The model under review builds one solid part; all positions refer to its coordinate system, in mm. A direction names the side the tool comes from. Coordinates: 2 decimals unless noted, no trailing zeros. Write each loop counter-clockwise with the first axis right and the second up, starting at its lowest first coordinate (ties: lowest second). Pieces come first, ordered by that corner, then holes. Notation, with made-up numbers: (-23.5, 80) - (19.5, 80) arc R25 ccw to (19.5, 115) - close; hole circle Ø11 at (75, 80). An arc over 180 degrees is marked (long way). Use one line per item in the form item = value. Start each with the question number.
```python
from build123d import *

# Parameters (mm, degrees)
SKETCH1_W               = 58
SKETCH1_H               = 58
BOSS_EXTRUDE1_DEPTH     = 10
BOSS_EXTRUDE3_DEPTH     = 30.005
CIRPATTERN7_COUNT       = 4
CUT_EXTRUDE1_DEPTH      = 13
CUT_EXTRUDE1_DEPTH_BACK = 11
SKETCH8_R               = 1.75
CUT_EXTRUDE2_DEPTH      = 20
SKETCH9_R               = 3.665
CUT_EXTRUDE3_DEPTH      = 2.1


with BuildPart() as part:
    # Sketch1 → Boss-Extrude1 (new body)
    with BuildSketch(Plane(origin=(0, 0, 0), x_dir=(1, 0, 0), z_dir=(0, 1, 0))):
        Rectangle(SKETCH1_W, SKETCH1_H)
    extrude(amount=BOSS_EXTRUDE1_DEPTH)

    # Sketch2 → Boss-Extrude3 (add, symmetric)
    with BuildSketch(Plane.XY):
        with BuildLine():
            Line((29, 0), (29, 14))
            Line((29, 14), (40.244226325, 21.496150883))
            ThreePointArc((40.244226325, 21.496150883), (41.038974467, 21.871276079), (41.908326913, 22))
            Line((41.908326913, 22), (44, 22))
            Line((44, 22), (31, 0))
            Line((31, 0), (29, 0))
        make_face()
    boss_extrude3 = extrude(amount=BOSS_EXTRUDE3_DEPTH, both=True)

    # CirPattern7: Boss-Extrude3 ×4 about axis
    cirpattern7_axis = Axis((0, 0, 0), (0, 1, 0))
    for i in range(1, CIRPATTERN7_COUNT):
        add(boss_extrude3.rotate(cirpattern7_axis, i * 360 / CIRPATTERN7_COUNT))

    # Sketch7 → Cut-Extrude1 (cut, two sides)
    with BuildSketch(Plane(origin=(0, 10, 0), x_dir=(1, 0, 0), z_dir=(0, 1, 0))) as cut_extrude1_sk:
        with BuildLine():
            Line((21.84, 7), (54.527297937, 7))
            Line((54.527297937, 7), (54.527297937, -7))
            Line((54.527297937, -7), (21.84, -7))
            ThreePointArc((21.84, -7), (14.84, 0), (21.84, 7))
        make_face()
        with BuildLine():
            Line((7, -21.84), (7, -54.527297937))
            Line((7, -54.527297937), (-7, -54.527297937))
            Line((-7, -54.527297937), (-7, -21.84))
            ThreePointArc((-7, -21.84), (0, -14.84), (7, -21.84))
        make_face()
        with BuildLine():
            Line((-21.84, -7), (-54.527297937, -7))
            Line((-54.527297937, -7), (-54.527297937, 7))
            Line((-54.527297937, 7), (-21.84, 7))
            ThreePointArc((-21.84, 7), (-14.84, 0), (-21.84, -7))
        make_face()
        with BuildLine():
            Line((-7, 21.84), (-7, 54.527297937))
            Line((-7, 54.527297937), (7, 54.527297937))
            Line((7, 54.527297937), (7, 21.84))
            ThreePointArc((7, 21.84), (0, 14.84), (-7, 21.84))
        make_face()
    extrude(amount=CUT_EXTRUDE1_DEPTH, mode=Mode.SUBTRACT)
    extrude(cut_extrude1_sk.sketch, amount=-CUT_EXTRUDE1_DEPTH_BACK, mode=Mode.SUBTRACT)

    # Sketch8 → Cut-Extrude2 (cut)
    with BuildSketch(Plane(origin=(-225.294025085, 10, 60.777514946), x_dir=(0, 0, -1), z_dir=(0, 1, 0))):
        with Locations((74.91965057, -211.151889461)):
            Circle(SKETCH8_R)
        with Locations((74.91965057, -239.436160708)):
            Circle(SKETCH8_R)
        with Locations((46.635379323, -239.436160708)):
            Circle(SKETCH8_R)
    extrude(amount=-CUT_EXTRUDE2_DEPTH, mode=Mode.SUBTRACT)

    # Sketch9 → Cut-Extrude3 (cut)
    with BuildSketch(Plane(origin=(0, 10, 0), x_dir=(1, 0, 0), z_dir=(0, 1, 0))):
        with Locations((-14.142135624, 14.142135624)):
            Circle(SKETCH9_R)
        with Locations((14.142135624, -14.142135624)):
            Circle(SKETCH9_R)
        with Locations((14.142135624, 14.142135624)):
            Circle(SKETCH9_R)
    extrude(amount=-CUT_EXTRUDE3_DEPTH, mode=Mode.SUBTRACT)


solid = part.part
```
1. Take a section at A-A (z = 34.5). State the section outline as (x, y) points (3 decimals).
2. Take a section at B-B (x = 38.5). State the section outline as (y, z) points (3 decimals), plus the area to 3 significant figures.
3. For P1, Ø11, axis at x = -32.5, y = 16, coming from the -Z side; P2, Ø3, axis at x = -14.14, z = -14.14, coming from the -Y side; P3, Ø3, axis at x = -1, y = 3.5, coming from the +Z side; P4, Ø10, axis at x = 10, y = 6, coming from the -Z side, all flat-tipped, find the tip position at first contact; note any pin that passes through.
4. For faces 4 (the flat face through (30, 9, -7)), 5 (the cylindrical face through (16.112, 8.965, -17.232)), 6 (the flat face through (-37.59, 11.15, 18.34)), 7 (the flat face through (-7, 9, 31)), list the 3-axis set-ups (+Z, -Z, +X, -X, +Y, -Y) from which the entire face can be reached by the end or side of a thin tool; tool diameter is ignored.
5. For L1, parallel to X at y = 16.5, z = 38 (3 decimals); L2, parallel to X at y = 9.75, z = -14.5, list the stretches that pass through material, from the lowest coordinate up.
6. Take a section at C-C (y = 12.75). Count the separate pieces of the cut face and the enclosed holes in it, plus the area to 3 significant figures.
7. The part is to be moulded in two halves that separate along Z. For faces 1 (the flat face through (-36, 14, -30.005)), 2 (the cylindrical face through (-12.17, 8.96, -17.23)), 3 (the flat face through (7, 9, -31)), say which applies: released by +Z, released by -Z, zero draft, split by the parting line, or undercut.
Returned:
q1.outline = (-30.005, 5.923) - (-7, 5.923) - (-7, 17.667) - (-30.005, 17.667) - close; (7, 5.923) - (30.005, 5.923) - (30.005, 17.667) - (7, 17.667) - close
q2.outline = (12.692, -30.005) - (20.333, -30.005) - (20.333, -7) - (12.692, -7) - close; (12.692, 7) - (20.333, 7) - (20.333, 30.005) - (12.692, 30.005) - close
q2.area = 352 mm²
q3.P1 = -43.35
q3.P2 = through
q3.P3 = 15.3
q3.P4 = -37.5
q4.face_4 = +X, +Y, -Y
q4.face_5 = +Y
q4.face_6 = +Z, -Z, -X, -Y
q4.face_7 = +Z, +Y, -Y
q5.L1 = -30.005 to -7, 7 to 30.005
q5.L2 = -36.76 to -17.79, -10.49 to 10.49, 17.79 to 36.76
q6.separate_pieces = 4
q6.enclosed_holes = 0
q6.area = 1,750 mm²
q7.face_1 = released by -Z
q7.face_2 = undercut
q7.face_3 = zero draft
